from build123d import *

# Parameters (mm, degrees)
F0_R     = 17.5
F0_W     = 10
F0_H     = 30
F0_W_2   = 8
F0_H_2   = 15
F1_DEPTH = 25.4


with BuildPart() as f1:
    # F0 (on Top) → F1 (new body)
    with BuildSketch(Plane.XY):
        Polygon((96.7858138128, 1.0294117647), (96.7858138128, 26.0294117647), (-58.2141861872, 26.0294117647), (-58.2141861872, 1.0294117647), (-48.2141861872, 1.0294117647), (-38.2141861872, 1.0294117647), (-30.2141861872, 1.0294117647), (-20.2141861872, 1.0294117647), (-6.2141861872, 1.0294117647), align=None)
        with BuildLine():
            ThreePointArc((96.7858138128, 1.0294117647), (164.4775558894, 13.5294117647), (96.7858138128, 26.0294117647))
            Line((96.7858138128, 26.0294117647), (96.7858138128, 1.0294117647))
        make_face()
        with Locations((129.4775558894, 13.5294117647)):
            Circle(F0_R, mode=Mode.SUBTRACT)
        with Locations((129.4775558894, 13.5294117647)):
            Circle(F0_R)
        with Locations((-53.2141861872, -13.9705882353)):
            Rectangle(F0_W, F0_H)
        with Locations((-34.2141861872, -6.4705882353)):
            Rectangle(F0_W_2, F0_H_2)
        Polygon((-13.3046329277, -13.9705882353), (-6.2141861872, 1.0294117647), (-20.2141861872, 1.0294117647), align=None)
    extrude(amount=F1_DEPTH)


solid = f1.part
Work out the finished part from the listing and answer in its coordinate system (mm). A direction names the side the tool comes from. Give positions to 0.01 mm unless a question says otherwise; leave off trailing zeros. Write each loop counter-clockwise with the first axis right and the second up, starting at its lowest first coordinate (ties: lowest second). Pieces come first, ordered by that corner, then holes. Notation, with made-up numbers: M 32.25,54.25 L 66.25,54.25 A33 cw 66.25,84.25 Z; hole C 40,-10 d10. An arc over 180 degrees is marked long. Answer as CSV lines item,"result".
Q1. The mould has two halves that part along X. Classify faces 1 (the flat face through (76, 10, 25.4)), 2 (the flat face through (-58.214, -1, 13)), 3 (the flat face through (-34, -13.971, 13)): +X half, -X half, draft (parallel to the pull), parting line (faces both ways), or undercut.
A:
face 1,"draft"
face 2,"-X half"
face 3,"undercut"
Q2. A cutting plane is placed at B-B on z = 18. Write down the section's boundary in (x, y).
A:
outline,"M -58.21,-28.97 L -48.21,-28.97 L -48.21,1.03 L -38.21,1.03 L -38.21,-13.97 L -30.21,-13.97 L -30.21,1.03 L -20.21,1.03 L -13.3,-13.97 L -6.21,1.03 L 96.79,1.03 A35 ccw long 96.79,26.03 L -58.21,26.03 Z"
Q3. A cutting plane is placed at A-A on y = -10. Write down the section's boundary in (x, z), plus the area to 3 significant figures.
A:
outline,"M -58.21,0 L -48.21,0 L -48.21,25.4 L -58.21,25.4 Z; M -38.21,0 L -30.21,0 L -30.21,25.4 L -38.21,25.4 Z; M -15.13,0 L -11.43,0 L -11.43,25.4 L -15.13,25.4 Z; M 103.57,0 L 155.39,0 L 155.39,25.4 L 103.57,25.4 Z"
area,"1,870 mm²"
Q4. A cutting plane is placed at C-C on x = 45.5. Write down the section's boundary in (y, z), plus the area to 3 significant figures.
A:
outline,"M 1.03,0 L 26.03,0 L 26.03,25.4 L 1.03,25.4 Z"
area,"635 mm²"
Q5. Find the intervals of material crossed by probe 1 along X at (y, z) = (-0.5, 16); probe 2 along X at (y, z) = (-5, 23.5); probe 3 along Y at (x, z) = (-1, 1.75), in increasing order. Write a range as [from, to].
A:
probe 1,"x = [-58.21, -48.21], [-38.21, -30.21], [-19.51, -6.94], [97.41, 161.54]"
probe 2,"x = [-58.21, -48.21], [-38.21, -30.21], [-17.44, -9.06], [99.78, 159.17]"
probe 3,"y = [1.03, 26.03]"
Q6. A cutting plane is placed at D-D on y = 38.5. Write down the section's boundary in (x, z).
A:
outline,"M 104.95,0 L 154,0 L 154,25.4 L 104.95,25.4 Z"
Q7. A tool of negligible diameter and unlimited length cuts with its end or side. For faces 4 (the flat face through (20, 26.029, 13)), 5 (the flat face through (-43, 1.029, 13)), 6 (the flat face through (-53, -28.971, 13)), from which of +Z, -Z, +X, -X, +Y, -Y can it reach the whole face along a straight path? Write none if from no direction.
A:
face 4,"+Z, -Z, -X, +Y"
face 5,"+Z, -Z, -Y"
face 6,"+Z, -Z, +X, -X, -Y"
Q8. Given P1, Ø4, axis at x = 22, y = 21.5, coming from the -Z side; P2, Ø10, axis at y = -10.5, z = 4, coming from the +X side; P3, Ø3, axis at y = 35, z = 5.5, coming from the -X side; P4, Ø2.5, axis at x = -34.5, z = 18.5, coming from the -Y side, each flat-ended and moving along its own axis, determine where each tip first touches the part or whether it passes through.
A:
P1,"stops at z = 0"
P2,"stops at x = 158.85"
P3,"stops at x = 100.73"
P4,"stops at y = -13.97"
